Autodesk Inventor part; units mm, degrees
ref_plane "YZ Plane" through (0, 0, 0) normal (1, 0, 0) x (0, 1, 0)
ref_plane "XZ Plane" through (0, 0, 0) normal (0, 1, 0) x (-1, 0, 0)
ref_plane "XY Plane" through (0, 0, 0) normal (0, 0, 1) x (1, 0, 0)
sketch "Szkic1" plane through (0, 0, 0) normal (0, 0, 1) x (1, 0, 0)
  line L0 (-16.906, 7.7541) -> (43.094, 7.7541)
  line L1 (43.094, 7.7541) -> (43.094, -2.2459)
  line L2 (43.094, -2.2459) -> (-16.906, -2.2459)
  line L3 (-16.906, -2.2459) -> (-16.906, 7.7541)
  arc A0 (-16.906, 7.7541) -> (-16.906, -2.2459) centre (-16.906, 2.7541) ccw
  circle A1 centre (-16.906, 2.7541) radius 3
  point P0 (0, 0)
  dimension "d0" = 60
  dimension "d1" = 10
  dimension "d2" = 6
extrude "Wyciągnięcie proste1" add sketch "Szkic1" along normal blind 10 contours L0 L1 L2 L3 A1 | L3 A1 A0
sketch "Szkic2" plane through (-16.906, -2.2459, 0) normal (0, -1, 0) x (1, 0, 0)
  line L0 (0, 0) -> (0, 10)
  line L1 (0, 5) -> (-8.6821, 5)
  line L2 (-8.6821, 5) -> (9.8833, 5)
  line L3 (-5, 0) -> (-5, 10)
  line L4 (-5, 7) -> (6, 7)
  line L5 (6, 7) -> (6, 3)
  line L6 (6, 3) -> (-5, 3)
  line L7 (-5, 3) -> (-5, 7)
  point P0 (16.906, 0)
  dimension "d5" = 11
  dimension "d6" = 4
extrude "Wyciągnięcie proste2" cut sketch "Szkic2" against normal blind 10
sketch "Szkic3" plane through (-16.906, -2.2459, 0) normal (0, -1, 0) x (1, 0, 0)
  line L0 (0, 10) -> (60, 10)
  line L1 (8, 10) -> (8, 0)
  line L2 (6, 7) -> (6, 3)
  line L3 (13, 7.5) -> (8, 7.5)
  line L4 (8, 7.5) -> (8, 2.5)
  line L5 (8, 2.5) -> (13, 2.5)
  line L6 (13, 2.5) -> (13, 7.5)
  line L7 (6, 5) -> (16.5434, 5)
  point P0 (16.906, 0)
  dimension "d9" = 2
  dimension "d10" = 5
  dimension "d11" = 5
extrude "Wyciągnięcie proste3" cut sketch "Szkic3" against normal blind 10
sketch "Szkic4" plane through (-16.906, -2.2459, 0) normal (0, -1, 0) x (1, 0, 0)
  line L0 (60, 0) -> (60, 10)
  line L1 (60, 10) -> (16, 10)
  line L2 (16, 10) -> (16, 8)
  line L3 (16, 8) -> (60, 8)
  line L4 (60, 8) -> (60, 10)
  line L5 (60, 0) -> (0, 0)
  line L6 (60, 0) -> (16, 0)
  line L7 (16, 0) -> (16, 2)
  line L8 (16, 2) -> (60, 2)
  line L9 (60, 2) -> (60, 0)
  point P0 (16.906, 0)
  point P1 (16, 0)
  dimension "d14" = 44
  dimension "d15" = 2
  dimension "d16" = 44
  dimension "d17" = 2
extrude "Wyciągnięcie proste4" cut sketch "Szkic4" against normal blind 10
sketch "Szkic5" plane through (-16.906, -2.2459, 7) normal (0, -1, 0) x (1, 0, 0)
  line L0 (16, 1) -> (60, 1)
  line L1 (30, 1) -> (30, -5.0068)
  line L2 (60, -5) -> (60, 1)
  line L3 (55, 1) -> (55, -5)
  line L4 (35, 1) -> (35, -5)
  line L5 (60, -5) -> (16, -5)
  line L6 (60, -2) -> (30, -2.0034)
  point P0 (16.906, -7)
  point P1 (55, -2.0006)
  point P2 (35, -2.0028)
  dimension "d20" = 30
  dimension "d21" = 5
  dimension "d22" = 25
hole "Otwór1" at (38.094, -2.2459, 4.9994) at (18.094, -2.2459, 4.9972) direction (0, 1, 0) diameter 2.459 end through all
properties part number "ramie" material "Stal nierdzewna 440C"
Geometry check sheet. Reference: the model listing, model coordinates, mm. A direction names the side the tool comes from. Round coordinates to 2 decimals unless told otherwise and drop trailing zeros. Loops run counter-clockwise (first coordinate to the right, second up) from the corner with the lowest first, then second, coordinate; pieces in that order, holes last. Notation, with made-up numbers: (52, 60) - (103, 60) arc R13 cw to (103, 77) - close; hole circle Ø2 at (83.25, 7). An arc over 180 degrees is marked (long way). One line per question, with ' | ' between items. Start each with the question number.
1. Cross-section at B-B on x = -13. Record the cut outline in (y, z), then the cut area to 3 significant figures.
2. Cross-section at C-C on z = 4.75. Record the cut outline in (x, y), then the cut area to 3 significant figures.
3. Draft check along X on faces 1 (the face through (43.094, 3, 5)), 2 (the face through (-9, 3, 10)), 3 (the face through (-3.906, 3, 5)), 4 (the face through (37.057, 2.824, 4.338)). Enter one of: released by +X, released by -X, zero draft, split by the parting line, or undercut.
4. Depth check by flat-ended pin: pin 1 (3 mm diameter, centred on y = 5, z = 6, fed in from -X); pin 2 (5 mm diameter, centred on x = -16.91, y = 2.75, fed in from -Z); pin 3 (6 mm diameter, centred on y = 4.5, z = 6.5, fed in from -X); pin 4 (1.5 mm diameter, centred on y = 5.5, z = 8, fed in from -X). Enter the tip coordinate at first touch or a pass-through.
5. Cross-section at A-A on y = 4.5. Record the cut outline in (x, z).
6. Tool access check on faces 5 (the face through (-0.906, 3, 1)), 6 (the face through (-14, 4, 7)), 7 (the face through (-6, 3, 2.5)). Record the directions out of +Z, -Z, +X, -X, +Y, -Y that give a thin tool (end or side, any length) a straight path to the whole face; none if there is none.
7. Cross-section at D-D on y = -1. Record the cut outline in (x, z), then the cut area to 3 significant figures.
8. Scan lines: line 1 (X direction, y = 2, z = 5); line 2 (Y direction, x = -17, z = 2.25); line 3 (Z direction, x = -16.5, y = -1.5). Record each from-to range of solid material in increasing order. Write a range as [from, to].
Taken from the geometry:
1) outline: (-2.25, 0) - (7.75, 0) - (7.75, 3) - (-2.25, 3) - close; (-2.25, 7) - (7.75, 7) - (7.75, 10) - (-2.25, 10) - close | area: 60.0 mm²
2) outline: (-10.91, -2.25) - (-8.91, -2.25) - (-8.91, 7.75) - (-10.91, 7.75) - close; (-3.91, -2.25) - (16.89, -2.25) - (16.89, 7.75) - (-3.91, 7.75) - close; (19.3, -2.25) - (36.89, -2.25) - (36.89, 7.75) - (19.3, 7.75) - close; (39.3, -2.25) - (43.09, -2.25) - (43.09, 7.75) - (39.3, 7.75) - close | area: 442 mm²
3) face 1: released by +X | face 2: zero draft | face 3: undercut | face 4: undercut
4) pin 1: x = -21.78 | pin 2: through | pin 3: x = -21.91 | pin 4: x = -21.49
5) outline: (-21.59, 0) - (-19.35, 0) - (-19.35, 3) - (-21.59, 3) - close; (-21.59, 7) - (-19.35, 7) - (-19.35, 10) - (-21.59, 10) - close; (-14.47, 0) - (-0.91, 0) - (-0.91, 2) - (43.09, 2) - (43.09, 8) - (-0.91, 8) - (-0.91, 10) - (-14.47, 10) - (-14.47, 7) - (-10.91, 7) - (-10.91, 3) - (-14.47, 3) - close; hole (-8.91, 2.5) - (-3.91, 2.5) - (-3.91, 7.5) - (-8.91, 7.5) - close; hole circle Ø2.46 at (18.09, 5); hole circle Ø2.46 at (38.09, 5)
6) face 5: -Z, +X, +Y, -Y | face 6: -X, +Y, -Y | face 7: +Y, -Y
7) outline: (-20.21, 0) - (-0.91, 0) - (-0.91, 2) - (43.09, 2) - (43.09, 8) - (-0.91, 8) - (-0.91, 10) - (-20.21, 10) - (-20.21, 7) - (-10.91, 7) - (-10.91, 3) - (-20.21, 3) - close; hole (-8.91, 2.5) - (-3.91, 2.5) - (-3.91, 7.5) - (-8.91, 7.5) - close; hole circle Ø2.46 at (18.09, 5); hole circle Ø2.46 at (38.09, 5) | area: 385 mm²
8) line 1: [-10.91, -8.91], [-3.91, 16.86], [19.32, 36.86], [39.32, 43.09] | line 2: [-2.25, -0.24], [5.75, 7.75] | line 3: [0, 3], [7, 10]
